Build history of the part. All positions in model axes, mm. Round coordinates to 2 decimals unless told otherwise and drop trailing zeros. Write each loop counter-clockwise with the first axis right and the second up, starting at its lowest first coordinate (ties: lowest second). Pieces come first, ordered by that corner, then holes. Notation, with made-up numbers: M 15,36.25 L 53,36.25 A19 ccw 53,46.25 Z; hole C 54.25,63 d10. An arc over 180 degrees is marked long. Write item = value, one per line. Start each with the question number.
Q1. Band-saw the part on B-B on x = 88.5. Write the cut outline in (y, z) (3 decimals), plus the area to 3 significant figures.
Q2. Drop a flat-ended pin along its axis: P1, Ø3.5, axis at x = -11.51, y = 5.22, coming from the +Z side. Give the stop position or say it passes through.
Q3. Probe L1, parallel to Y at x = -37.5, z = 1.3 (1 decimal); L2, parallel to Y at x = -85, z = 2 (3 decimals); L3, parallel to Y at x = -190, z = 0.45 (3 decimals). List the from-to ranges inside material, lowest first.
Q4. Band-saw the part on C-C on z = 1.3. State how many separate pieces and enclosed holes the cut face has, plus the area to 3 significant figures.
Q5. Band-saw the part on A-A on x = 191. Write the cut outline in (y, z) (3 decimals), plus the area to 3 significant figures.
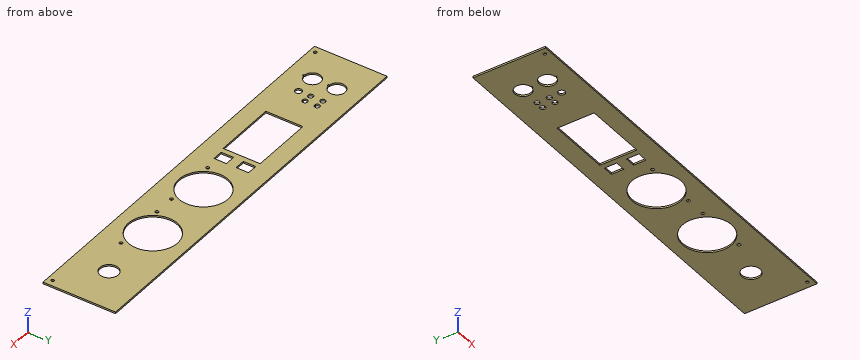
```python
from build123d import *

# Parameters (mm, degrees)
SKETCH1_W              = 482.6
SKETCH1_H              = 88.9
FRONT_PANEL_DEPTH      = 2.1
MOUNTING_HOLES_REACH   = 252.351
SKETCH7_R              = 1.89865
START_STOP_DEPTH       = 251.351064757
SKETCH3_R              = 3.175
MODE_SELECT_DEPTH      = 251.351064757
SKETCH4_W              = 76
SKETCH4_H              = 45.5
LCD_CUTOUT_DEPTH       = 251.351064757
SKETCH5_R              = 11.25
E_STOP_CUTOUT_DEPTH    = 251.351064757
SKETCH6_W              = 12.7
SKETCH6_H              = 15.24
LCD_PUSHBUTTONS_DEPTH  = 251.351064757
ERROR_INDICATOR_REACH  = 252.351
SKETCH8_R              = 4.15
PANEL_METER_CUTOUT_R   = 30
PANEL_METER_CUTOUT_R_2 = 2
PANEL_METER_DEPTH      = 251.351064757
LPATTERN1_COUNT        = 2
LPATTERN1_PITCH        = 90


with BuildPart() as part:
    # Sketch1 → Front panel (new body)
    with BuildSketch(Plane.XY):
        with Locations((0, 22.225)):
            Rectangle(SKETCH1_W, SKETCH1_H)
    extrude(amount=FRONT_PANEL_DEPTH)

    # Sketch7 → Mounting holes (cut, up to next)
    with BuildSketch(Plane.XY.offset(2.1), mode=Mode.PRIVATE) as mounting_holes_sk1:
        with Locations((-233.3625, -15.875)):
            Circle(SKETCH7_R)
    mounting_holes_tool1 = extrude(mounting_holes_sk1.sketch, amount=-MOUNTING_HOLES_REACH, mode=Mode.PRIVATE) & part.part
    # Sketch7 → Mounting holes (cut, up to next)
    with BuildSketch(Plane.XY.offset(2.1), mode=Mode.PRIVATE) as mounting_holes_sk2:
        with Locations((233.3625, -15.875)):
            Circle(SKETCH7_R)
    mounting_holes_tool2 = extrude(mounting_holes_sk2.sketch, amount=-MOUNTING_HOLES_REACH, mode=Mode.PRIVATE) & part.part
    add(mounting_holes_tool1.solids().sort_by_distance((-233.3625, -15.875, 2.1))[0], mode=Mode.SUBTRACT)
    add(mounting_holes_tool2.solids().sort_by_distance((233.3625, -15.875, 2.1))[0], mode=Mode.SUBTRACT)

    # Sketch2 → Start/stop (cut, through all)
    with BuildSketch(Plane.XY.offset(2.1)):
        with BuildLine():
            Line((-196.175880429, 27.185079682), (-196.175880429, 25.725))
            Line((-196.175880429, 25.725), (-193.975880429, 25.725))
            Line((-193.975880429, 25.725), (-193.975880429, 27.185079682))
            ThreePointArc((-193.975880429, 27.185079682), (-195.075880429, 47.325), (-196.175880429, 27.185079682))
        make_face()
        with BuildLine():
            Line((-196.175880429, -2.814920318), (-196.175880429, -4.275))
            Line((-196.175880429, -4.275), (-193.975880429, -4.275))
            Line((-193.975880429, -4.275), (-193.975880429, -2.814920318))
            ThreePointArc((-193.975880429, -2.814920318), (-195.075880429, 17.325), (-196.175880429, -2.814920318))
        make_face()
    extrude(amount=-START_STOP_DEPTH, mode=Mode.SUBTRACT)

    # Sketch3 → Mode select (cut, through all)
    with BuildSketch(Plane.XY.offset(2.1)):
        with Locations((-170.075880429, 37.225)):
            Circle(SKETCH3_R)
        with Locations((-170.075880429, 22.225)):
            Circle(SKETCH3_R)
        with BuildLine():
            Line((-160.375880429, 33.988875775), (-160.375880429, 34.875))
            Line((-160.375880429, 34.875), (-159.775880429, 34.875))
            Line((-159.775880429, 34.875), (-159.775880429, 33.988875775))
            ThreePointArc((-159.775880429, 33.988875775), (-160.075880429, 40.475), (-160.375880429, 33.988875775))
        make_face()
        with BuildLine():
            Line((-160.375880429, 18.988875775), (-160.375880429, 19.875))
            Line((-160.375880429, 19.875), (-159.775880429, 19.875))
            Line((-159.775880429, 19.875), (-159.775880429, 18.988875775))
            ThreePointArc((-159.775880429, 18.988875775), (-160.075880429, 25.475), (-160.375880429, 18.988875775))
        make_face()
    extrude(amount=-MODE_SELECT_DEPTH, mode=Mode.SUBTRACT)

    # Sketch4 → LCD cutout (cut, through all)
    with BuildSketch(Plane.XY.offset(2.1)):
        with Locations((-85.340826022, 22.225)):
            Rectangle(SKETCH4_W, SKETCH4_H)
    extrude(amount=-LCD_CUTOUT_DEPTH, mode=Mode.SUBTRACT)

    # Sketch5 → E-stop cutout (cut, through all)
    with BuildSketch(Plane.XY.offset(2.1)):
        with Locations((188.308959836, 22.225)):
            Circle(SKETCH5_R)
    extrude(amount=-E_STOP_CUTOUT_DEPTH, mode=Mode.SUBTRACT)

    # Sketch6 → LCD pushbuttons (cut, through all)
    with BuildSketch(Plane.XY.offset(2.1)):
        with Locations((-34.530826022, 36.3075)):
            Rectangle(SKETCH6_W, SKETCH6_H)
        with Locations((-34.530826022, 9.19)):
            Rectangle(SKETCH6_W, SKETCH6_H)
    extrude(amount=-LCD_PUSHBUTTONS_DEPTH, mode=Mode.SUBTRACT)

    # Sketch8 → ERROR indicator (cut, up to next)
    with BuildSketch(Plane.XY.offset(2.1), mode=Mode.PRIVATE) as error_indicator_sk1:
        with Locations((-170.075880429, 7.225)):
            Circle(SKETCH8_R)
    error_indicator_tool1 = extrude(error_indicator_sk1.sketch, amount=-ERROR_INDICATOR_REACH, mode=Mode.PRIVATE) & part.part
    add(error_indicator_tool1.solids().sort_by_distance((-170.07588, 7.225, 2.1))[0], mode=Mode.SUBTRACT)

    # Panel meter cutout → Panel meter (cut, through all)
    with BuildSketch(Plane.XY.offset(2.1)):
        with Locations((20.488631919, 22.225)):
            Circle(PANEL_METER_CUTOUT_R)
        with Locations((52.488631919, 5.225)):
            Circle(PANEL_METER_CUTOUT_R_2)
        with Locations((-11.511368081, 5.225)):
            Circle(PANEL_METER_CUTOUT_R_2)
    panel_meter = extrude(amount=-PANEL_METER_DEPTH, mode=Mode.SUBTRACT)

    # LPattern1: Panel meter ×2
    with Locations(*[(i * LPATTERN1_PITCH, 0, 0) for i in range(1, LPATTERN1_COUNT)]):
        add(panel_meter, mode=Mode.SUBTRACT)


solid = part.part
```
Conclusion:
q1.outline = M -22.225,0 L 1.817,0 L 1.817,2.1 L -22.225,2.1 Z; M 42.633,0 L 66.675,0 L 66.675,2.1 L 42.633,2.1 Z
q1.area = 101 mm^2
q2.P1 = through
q3.L1 = -22.2 to 1.6, 16.8 to 28.7, 43.9 to 66.7
q3.L2 = -22.225 to -0.525, 44.975 to 66.675
q3.L3 = -22.225 to -1.507, 15.957 to 28.493, 45.957 to 66.675
q4.separate_pieces = 1
q4.enclosed_holes = 19
q4.area = 32,100 mm^2
q5.outline = M -22.225,0 L 11.302,0 L 11.302,2.1 L -22.225,2.1 Z; M 33.148,0 L 66.675,0 L 66.675,2.1 L 33.148,2.1 Z
q5.area = 141 mm^2
